from build123d import *

# Parameters (mm, degrees)
F0_W     = 55.7806007564
F0_H     = 58.5907548666
F0_R     = 15.6812666629
F1_DEPTH = 25.4
F3_DEPTH = 25
F4_DEPTH = 25


with BuildPart() as f1:
    # F0 (on Top) → F1 (new body)
    with BuildSketch(Plane.XY):
        with Locations((-0.8635763079, 0.0774934888)):
            Rectangle(F0_W, F0_H)
        Circle(F0_R, mode=Mode.SUBTRACT)
    extrude(amount=F1_DEPTH)

    # F2 (on Top) → F3 (join)
    with BuildSketch(Plane.XY):
        Polygon((-46.4129857719, -45.5937832594), (46.0013560951, -46.0371151567), (46.0013560951, 45.8016321063), (-46.4129857719, 45.8016321063), align=None)
    extrude(amount=F3_DEPTH)

    # F4 (add): faces of the model
    f4_faces = [f1.faces().sort_by_distance(p)[0] for p in [
        (26.2177523788, 0.0774934888, 25.4),
        (-0.199564745, -44.5125917544, 25),
    ]]
    extrude(f4_faces, amount=F4_DEPTH)


solid = f1.part
Can you work these out from the model? Positions are in its coordinate system, mm. A direction names the side the tool comes from. Give positions to 0.01 mm unless a question says otherwise; leave off trailing zeros. Loops run counter-clockwise (first coordinate to the right, second up) from the corner with the lowest first, then second, coordinate; pieces in that order, holes last. Notation, with made-up numbers: (-31.75, -28.5) -> (3.25, -28.5) arc R15 ccw to (3.25, 0.5) -> close; hole circle Ø8 at (71, 42.5). An arc over 180 degrees is marked (long way). Return JSON: item names as keys, results as strings.
Q1. I want a section at A-A, the plane z = 47. List the corners of the cut face in (x, y) for me.
Checks:
{"outline": "(-46.41, -45.59) -> (46, -46.04) -> (46, 45.8) -> (-46.41, 45.8) -> close; hole circle Ø31.36 at (0, 0)"}
Q2. I want a section at C-C, the plane x = 9. List the corners of the cut face in (y, z) for me, then the cut area to 3 significant figures.
Checks:
{"outline": "(-45.86, 0) -> (45.8, 0) -> (45.8, 50) -> (29.37, 50) -> (29.37, 50.4) -> (12.84, 50.4) -> (12.84, 25) -> (-12.84, 25) -> (-12.84, 50.4) -> (-29.22, 50.4) -> (-29.22, 50) -> (-45.86, 50) -> close", "area": "3,950 mm2"}
Q3. I want a section at B-B, the plane y = -8.5. List the corners of the cut face in (x, z) for me.
Checks:
{"outline": "(-46.41, 0) -> (46, 0) -> (46, 50) -> (27.03, 50) -> (27.03, 50.4) -> (13.18, 50.4) -> (13.18, 25) -> (-13.18, 25) -> (-13.18, 50.4) -> (-28.75, 50.4) -> (-28.75, 50) -> (-46.41, 50) -> close"}
Q4. For pin 1 Ø8 at (x, z) = (-7.5, 38) entering from -Y, with a flat end and sliding along its axis, tell me the tip position at first contact or that it passes through.
Checks:
{"pin 1": "stops at y = -45.8"}
Q5. On a 3-axis mill with a long thin cutter (end or side, diameter ignored), from which of +Z, -Z, +X, -X, +Y, -Y can I reach the whole of each face in a straight line? I mean faces 1 (the face through (46.001, -1, 25)), 2 (the face through (14.957, 4.71, 37.522)). Say none if no direction works.
Checks:
{"face 1": "+Z, -Z, +X, +Y, -Y", "face 2": "+Z"}
Q6. I need wall thicknesses on probe 1 along X at (y, z) = (0, 36.5); probe 2 along Z at (x, y) = (34, 20.5); probe 3 along Y at (x, z) = (-1, 31). Which ranges of each line are inside material? Lowest first, please.
Checks:
{"probe 1": "x = -46.41 to -15.68, 15.68 to 46", "probe 2": "z = 0 to 50", "probe 3": "y = -45.81 to -15.65, 15.65 to 45.8"}
